from build123d import *

# Parameters (mm, degrees)
EXTRUDE_1_DEPTH     = 53
SKETCH_3_R          = 5
CUT_EXTRUDE_1_DEPTH = 75.01351228


with BuildPart() as part:
    # 草图1 → 凸台-拉伸1 (new, symmetric)
    with BuildSketch(Plane.XY):
        with BuildLine():
            Line((0, 1), (0, 37))
            ThreePointArc((0, 37), (0.292893219, 37.707106781), (1, 38))
            Line((1, 38), (2, 38))
            ThreePointArc((2, 38), (2.707106781, 37.707106781), (3, 37))
            Line((3, 37), (3, 8))
            ThreePointArc((3, 8), (4.464466094, 4.464466094), (8, 3))
            Line((8, 3), (37, 3))
            ThreePointArc((37, 3), (37.707106781, 2.707106781), (38, 2))
            Line((38, 2), (38, 1))
            ThreePointArc((38, 1), (37.707106781, 0.292893219), (37, 0))
            Line((37, 0), (1, 0))
            ThreePointArc((1, 0), (0.292893219, 0.292893219), (0, 1))
        make_face()
    extrude(amount=EXTRUDE_1_DEPTH, both=True)

    # 草图3 → 切除-拉伸1 (cut, through all)
    with BuildSketch(Plane(origin=(0, 3, 0), x_dir=(1, 0, 0), z_dir=(0, 1, 0))):
        with Locations(Location((21, 30.5, 0), (0, 0, 270))):
            Circle(SKETCH_3_R)
        with Locations(Location((21, -30.5, 0), (0, 0, 270))):
            Circle(SKETCH_3_R)
    extrude(amount=-CUT_EXTRUDE_1_DEPTH, mode=Mode.SUBTRACT)


solid = part.part
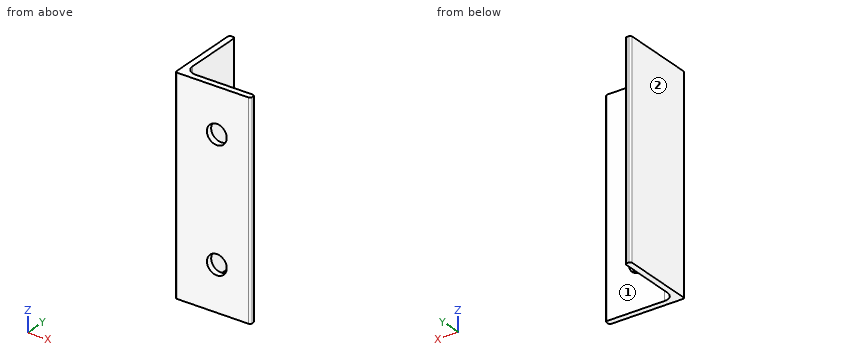
Build history of the part. All positions in model axes, mm. Face numbers are marked on the shaded views. A direction names the side the tool comes from. Give positions to 0.01 mm unless a question says otherwise; leave off trailing zeros. Order: outer loops, then holes, each group sorted by start corner. A loop starts at its lowest first (then second) coordinate and runs counter-clockwise, first axis right, second up. Notation, with made-up numbers: M 9,-8 L 48,-8 A15 ccw 48,11 Z; hole C 25,-7 d3. An arc over 180 degrees is marked long. Use one line per item in the form item = value.
Q1. Slice it at A-A, the plane x = 21. Write the cut outline in (y, z).
Conclusion:
outline = M 0,-53 L 3,-53 L 3,-35.5 L 0,-35.5 Z; M 0,-25.5 L 3,-25.5 L 3,25.5 L 0,25.5 Z; M 0,35.5 L 3,35.5 L 3,53 L 0,53 Z
Q2. Pin check, flat tips, straight feed: P1, Ø11.5, axis at x = 21, z = 30.5, coming from the +Y side; P2, Ø1.5, axis at y = 34, z = 37, coming from the +X side. Stop position of each tip, or through.
Conclusion:
P1 = 3
P2 = 3
Q3. Which spindle directions (+Z, -Z, +X, -X, +Y, -Y) get a long thin tool onto all of the face, cutting with end or side? Do the marked faces 1 and 2. Say none if no direction does.
Conclusion:
face_1 = +Z, -Z, +X, +Y
face_2 = +Z, -Z, -X, +Y, -Y
Q4. Slice it at D-D, the plane x = 5. Write the cut outline in (y, z).
Conclusion:
outline = M 0,-53 L 4,-53 L 4,53 L 0,53 Z
Q5. Wall check: probe 1 along X at (y, z) = (1.2, -30.5); probe 2 along X at (y, z) = (26.5, 42); probe 3 along X at (y, z) = (2.4, -30.5). Give the ranges that are in metal, low to high.
Conclusion:
probe_1 = 0 to 16, 26 to 38
probe_2 = 0 to 3
probe_3 = 0 to 16, 26 to 37.92
Q6. Slice it at B-B, the plane z = 30.5. Write the cut outline in (x, y).
Conclusion:
outline = M 0,1 A1 ccw 1,0 L 16,0 L 16,3 L 8,3 A5 cw 3,8 L 3,37 A1 ccw 2,38 L 1,38 A1 ccw 0,37 Z; M 26,0 L 37,0 A1 ccw 38,1 L 38,2 A1 ccw 37,3 L 26,3 Z
Q7. Slice it at C-C, the plane z = 46.5. Write the cut outline in (x, y).
Conclusion:
outline = M 0,1 A1 ccw 1,0 L 37,0 A1 ccw 38,1 L 38,2 A1 ccw 37,3 L 8,3 A5 cw 3,8 L 3,37 A1 ccw 2,38 L 1,38 A1 ccw 0,37 Z
